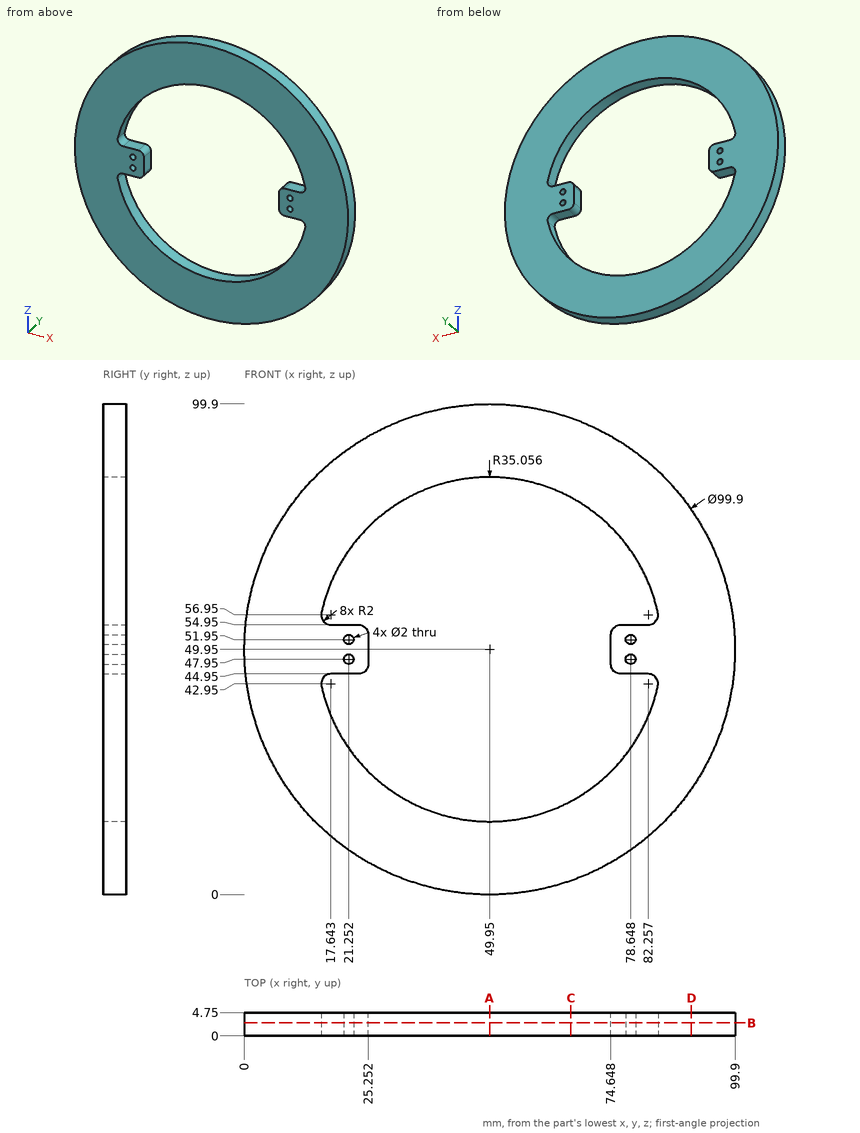
Can you work these out from the drawing? Everything is in mm from the part's minimum corner. Round coordinates to 2 decimals unless told otherwise and drop trailing zeros. Order: outer loops, then holes, each group sorted by start corner. A loop starts at its lowest first (then second) coordinate and runs counter-clockwise, first axis right, second up. Notation, with made-up numbers: (9, -5.5) -> (52, -5.5) arc R24 cw to (52, 11.5) -> close; hole circle Ø7 at (-15.5, 85.25). An arc over 180 degrees is marked (long way). Return JSON: item names as keys, results as strings. Group by question number.
1. If we section it at B-B, the plane y = 2.65: Write out the boundary of the cut face in (x, z).
2. If we section it at C-C, the plane x = 66.5: Write out the boundary of the cut face in (y, z), then the cut area to 3 significant figures.
3. If we section it at A-A, the plane x = 49.95: Write out the boundary of the cut face in (y, z).
4. If we section it at D-D, the plane x = 91: Write out the boundary of the cut face in (y, z).
5. Will these pins go through, and if not, where does the flat tip stop? pin 1 (2.5 mm diameter, centred on x = 21.5, y = 2, fed in from -Z) (1 decimal); pin 2 (2.5 mm diameter, centred on x = 21.25, z = 47.95, fed in from +Y); pin 3 (1.5 mm diameter, centred on x = 61, y = 2, fed in from +Z); pin 4 (1.4 mm diameter, centred on y = 3, z = 49.5, fed in from +X).
6. I need wall thicknesses on line 1 (X direction, y = 1.4, z = 47.95); line 2 (X direction, y = 2.7, z = 21.5) (1 decimal); line 3 (Z direction, x = 26.5, y = 4.55) (1 decimal). Which ranges of each line are inside material? Lowest first, please. Write a range as [from, to].
Output values:
{
 "1": {"outline": "circle Ø99.9 at (49.95, 49.95); hole (15.69, 42.53) arc R35.06 ccw to (84.21, 42.53) arc R2 ccw to (82.26, 44.95) -> (76.65, 44.95) arc R2 cw to (74.65, 46.95) -> (74.65, 52.95) arc R2 cw to (76.65, 54.95) -> (82.26, 54.95) arc R2 ccw to (84.21, 57.37) arc R35.06 ccw to (15.69, 57.37) arc R2 ccw to (17.64, 54.95) -> (23.25, 54.95) arc R2 cw to (25.25, 52.95) -> (25.25, 46.95) arc R2 cw to (23.25, 44.95) -> (17.64, 44.95) arc R2 ccw to start; hole circle Ø2 at (21.25, 47.95); hole circle Ø2 at (21.25, 51.95); hole circle Ø2 at (78.65, 47.95); hole circle Ø2 at (78.65, 51.95)"},
 "2": {"outline": "(0, 2.82) -> (4.75, 2.82) -> (4.75, 19.05) -> (0, 19.05) -> close; (0, 80.85) -> (4.75, 80.85) -> (4.75, 97.08) -> (0, 97.08) -> close", "area": "154 mm²"},
 "3": {"outline": "(0, 0) -> (4.75, 0) -> (4.75, 14.89) -> (0, 14.89) -> close; (0, 85.01) -> (4.75, 85.01) -> (4.75, 99.9) -> (0, 99.9) -> close"},
 "4": {"outline": "(0, 21.49) -> (4.75, 21.49) -> (4.75, 78.41) -> (0, 78.41) -> close"},
 "5": {"pin 1": "z = 8.1", "pin 2": "y = 4.75", "pin 3": "z = 98.83", "pin 4": "x = 99.9"},
 "6": {"line 1": "[0.04, 20.25], [22.25, 25.25], [74.65, 77.65], [79.65, 99.86]", "line 2": "[8.9, 29.5], [70.4, 91]", "line 3": "[5.8, 23.9], [76, 94.1]"}
}
